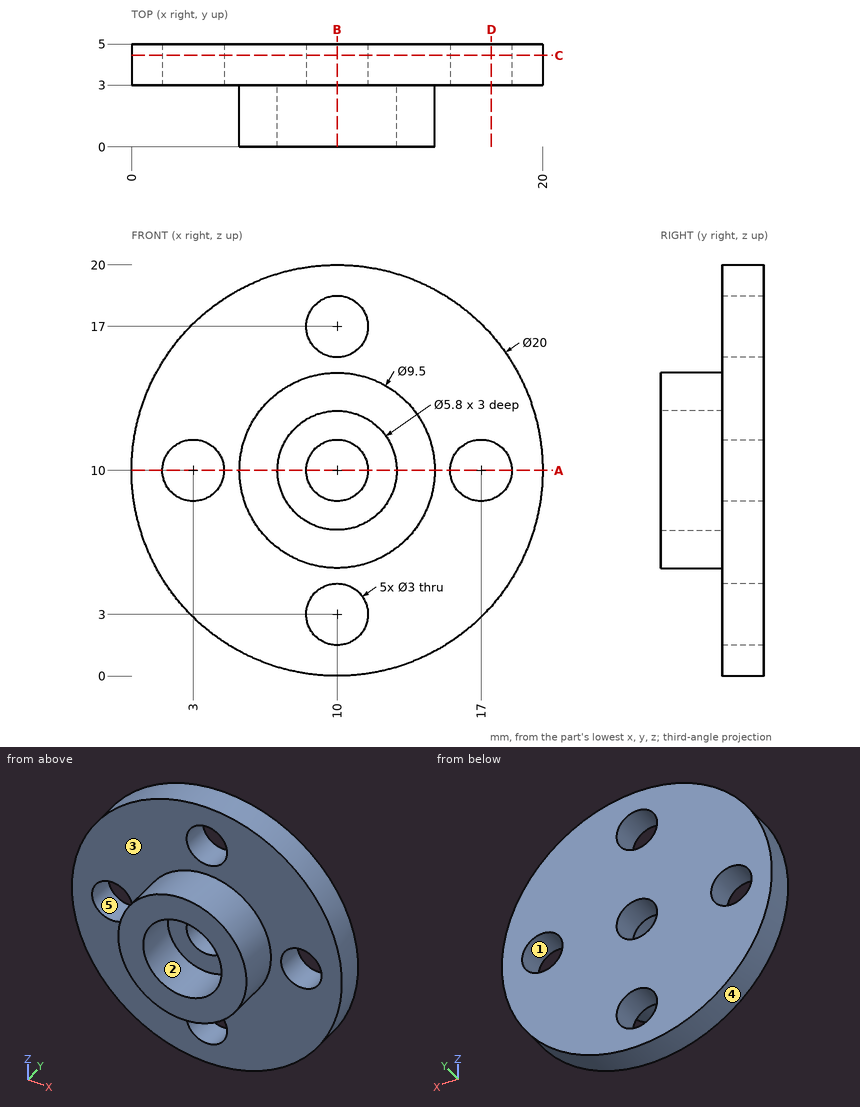
The figure shows three views and two pictorial views of one solid part (mm, origin at its lowest corner). Answer the questions. A direction names the side the tool comes from. Round coordinates to 2 decimals unless told otherwise and drop trailing zeros. Order: outer loops, then holes, each group sorted by start corner. A loop starts at its lowest first (then second) coordinate and runs counter-clockwise, first axis right, second up. Notation, with made-up numbers: M 41.5,10 L 91.5,10 A20 ccw 91.5,22 Z; hole C 17.25,84 d11. An arc over 180 degrees is marked long. Answer in a Markdown table with one row per item. Add a question column.
1) Which of the six approach directions +Z, -Z, +X, -X, +Y, -Y give full straight-line access (tool end or side, diameter ignored) to the marked faces 1 and 2?
2) The part is cut by section A-A on z = 10. Determine the outline of the cut face in (x, y), plus the area to 3 significant figures.
3) Flat-ended cylindrical pins translate along their axes: pin 1 Ø1.7 at (x, z) = (10.5, 10) entering from -Y; pin 2 Ø3 at (y, z) = (1, 11.5) entering from -X; pin 3 Ø2 at (x, z) = (2.5, 15.5) entering from -Y. Find the tip coordinate at first contact, or state that the pin passes through.
4) Consider line 1 along X through (y, z) = (1, 10); line 2 along X through (y, z) = (4.1, 10); line 3 along Z through (x, y) = (10.75, 3.45). Determine where each line is inside the solid, lowest interval first. Write a range as from..to.
5) The part is cut by section C-C on y = 4.45. Determine the outline of the cut face in (x, z).
6) Determine the mould class of the marked faces 3, 4 and 5 for opening direction X: pulls with the +X half, pulls with the -X half, needs draft (parallel to the pull), parting line crosses it, or undercut.
7) The part is cut by section B-B on x = 10. Determine the outline of the cut face in (y, z).
8) The part is cut by section D-D on x = 17.5. Determine the outline of the cut face in (y, z), plus the area to 3 significant figures.
Findings below:
| question | item | result |
|---|---|---|
| 1 | face 1 | +Y, -Y |
| 1 | face 2 | -Y |
| 2 | outline | M 0,3 L 1.5,3 L 1.5,5 L 0,5 Z; M 4.5,3 L 5.25,3 L 5.25,0 L 7.1,0 L 7.1,3 L 8.5,3 L 8.5,5 L 4.5,5 Z; M 11.5,3 L 12.9,3 L 12.9,0 L 14.75,0 L 14.75,3 L 15.5,3 L 15.5,5 L 11.5,5 Z; M 18.5,3 L 20,3 L 20,5 L 18.5,5 Z |
| 2 | area | 33.1 mm² |
| 3 | pin 1 | passes through |
| 3 | pin 2 | stops at x = 5.25 |
| 3 | pin 3 | stops at y = 3 |
| 4 | line 1 | x = 5.25..7.1, 12.9..14.75 |
| 4 | line 2 | x = 0..1.5, 4.5..8.5, 11.5..15.5, 18.5..20 |
| 4 | line 3 | z = 0.03..1.7, 4.3..8.7, 11.3..15.7, 18.3..19.97 |
| 5 | outline | C 10,10 d20; hole C 3,10 d3; hole C 10,3 d3; hole C 10,10 d3; hole C 10,17 d3; hole C 17,10 d3 |
| 6 | face 3 | needs draft |
| 6 | face 4 | parting line crosses it |
| 6 | face 5 | undercut |
| 7 | outline | M 0,5.25 L 3,5.25 L 3,4.5 L 5,4.5 L 5,8.5 L 3,8.5 L 3,7.1 L 0,7.1 Z; M 0,12.9 L 3,12.9 L 3,11.5 L 5,11.5 L 5,15.5 L 3,15.5 L 3,14.75 L 0,14.75 Z; M 3,0 L 5,0 L 5,1.5 L 3,1.5 Z; M 3,18.5 L 5,18.5 L 5,20 L 3,20 Z |
| 8 | outline | M 3,3.39 L 5,3.39 L 5,8.59 L 3,8.59 Z; M 3,11.41 L 5,11.41 L 5,16.61 L 3,16.61 Z |
| 8 | area | 20.8 mm² |
